Can you work these out from the model? Positions are in its coordinate system, mm. Face numbers are marked on the shaded views. A direction names the side the tool comes from. Coordinates: 2 decimals unless noted, no trailing zeros. Loops run counter-clockwise (first coordinate to the right, second up) from the corner with the lowest first, then second, coordinate; pieces in that order, holes last. Notation, with made-up numbers: M 15.5,-33.75 L 48.5,-33.75 A20 cw 48.5,-24.75 Z; hole C 85.25,54.25 d4. An arc over 180 degrees is marked long. Answer as a JSON object with one key per item and string values. Group by question number.
Item 1: If I drill on line 1 (Z direction, x = 0, y = -0.3); line 2 (X direction, y = 1.55, z = 0), over which ranges is the centre line in solid material (lowest first)?
Item 2: We'd pull the mould along Z, two halves only. Please class the marked faces 1, 2, 3 and 4: +Z half, -Z half, draft (parallel to the pull), parting line (faces both ways), or undercut.
Item 3: Which directions (+Z, -Z, +X, -X, +Y, -Y) give clear straight access to the entire face, cutting with the end or side of a thin tool? Please do the marked faces 5 and 6.
Item 4: Suppose I cut it at D-D (y = -2.6). Write out the boundary of the cut face in (x, z).
Item 5: Suppose I cut it at A-A (z = 0). Write out the boundary of the cut face in (x, y).
Item 6: Suppose I cut it at C-C (y = -0.35). Write out the boundary of the cut face in (x, z).
Item 7: Suppose I cut it at B-B (x = 0). Write out the boundary of the cut face in (y, z).
Item 8: I'm going to push flat-ended pins straight in: pin 1 Ø2 at (y, z) = (-1.5, 5.5) entering from -X; pin 2 Ø1.5 at (x, y) = (1.5, -1) entering from +Z; pin 3 Ø3 at (y, z) = (0.5, -5) entering from +X; pin 4 Ø2.5 at (x, z) = (0, 0) entering from -Y. Where does each tip first touch, or does it pass through?
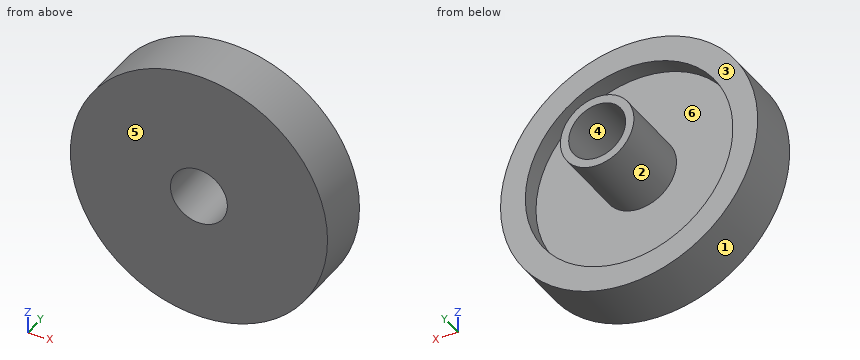
Autodesk Inventor part; units mm, degrees
ref_plane "YZ Plane" through (0, 0, 0) normal (1, 0, 0) x (0, 1, 0)
ref_plane "XZ Plane" through (0, 0, 0) normal (0, 1, 0) x (-1, 0, 0)
ref_plane "XY Plane" through (0, 0, 0) normal (0, 0, 1) x (1, 0, 0)
sketch "スケッチ1" plane through (0, 0, 0) normal (0, 0, 1) x (1, 0, 0)
  line L0 (1.55, 3) -> (1.55, -3)
  line L1 (1.55, -3) -> (7, -3)
  line L2 (7, -3) -> (7, 0)
  line L3 (7, 0) -> (2, 0)
  line L4 (2, 0) -> (2, 3)
  line L5 (2, 3) -> (1.55, 3)
  line L6 (0, -4.2) -> (0, 4.2)
  point P0 (0, 0)
  point P1 (1.55, 0)
  dimension "d0" = 1.55
  dimension "d1" = 2
  dimension "d2" = 3
  dimension "d3" = 7
  dimension "d4" = 3
revolve "回転1" add sketch "スケッチ1" angle 360 about axis through (0, -10, 0) along (0, 1, 0)
sketch "スケッチ2" plane through (0, 0, 0) normal (0, 1, 0) x (1, 0, 0)
  circle A0 centre (0, 0) radius 2
  circle A1 centre (0, 0) radius 7
  circle A2 centre (0, 0) radius 5.65
  dimension "d6" = 11.3
extrude "押し出し1" cut sketch "スケッチ2" against normal blind 1 contours A2
properties part number "付け根_サブフレーム_1_4" material "アセタール樹脂、黒"
From the geometry:
{
 "1": {"line 1": "-7 to -5.65, -2 to -1.55, 1.55 to 2, 5.65 to 7", "line 2": "-2 to -1.55, 1.55 to 2"},
 "2": {"face 1": "parting line", "face 2": "undercut", "face 3": "draft", "face 4": "undercut"},
 "3": {"face 5": "+Z, -Z, +X, -X, -Y", "face 6": "+Y"},
 "4": {"outline": "C 0,0 d14; hole C 0,0 d3.1"},
 "5": {"outline": "M -7,-3 L -1.55,-3 L -1.55,3 L -2,3 L -2,-1 L -5.65,-1 L -5.65,0 L -7,0 Z; M 1.55,-3 L 7,-3 L 7,0 L 5.65,0 L 5.65,-1 L 2,-1 L 2,3 L 1.55,3 Z"},
 "6": {"outline": "C 0,0 d14; C 0,0 d4; hole C 0,0 d11.3; hole C 0,0 d3.1"},
 "7": {"outline": "M -3,-7 L 0,-7 L 0,-5.65 L -1,-5.65 L -1,-2 L 3,-2 L 3,-1.55 L -3,-1.55 Z; M -3,1.55 L 3,1.55 L 3,2 L -1,2 L -1,5.65 L 0,5.65 L 0,7 L -3,7 Z"},
 "8": {"pin 1": "x = -5.36", "pin 2": "z = 6.96", "pin 3": "x = 6.01", "pin 4": "through"}
}
